For this review, take the finished solid that the model builds, in its own axes (mm). Face numbers are marked on the shaded views. A direction names the side the tool comes from. Round coordinates to 2 decimals unless told otherwise and drop trailing zeros. Order: outer loops, then holes, each group sorted by start corner. A loop starts at its lowest first (then second) coordinate and runs counter-clockwise, first axis right, second up. Notation, with made-up numbers: M 14,75 L 59,75 A27 cw 59,107 Z; hole C -5.5,7.5 d4. An arc over 180 degrees is marked long. Put each result on its own line as item: value.
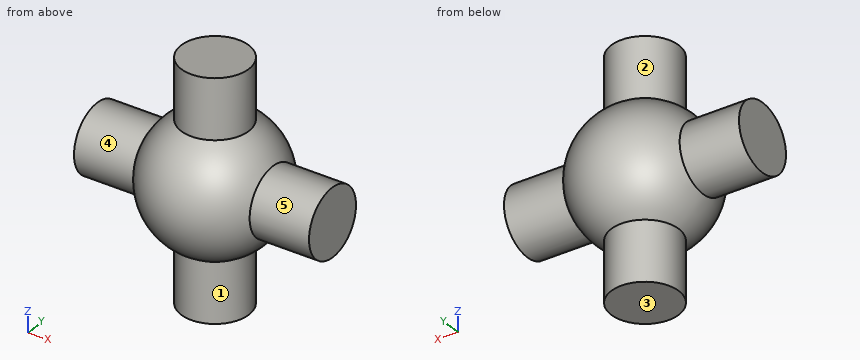
from build123d import *

# Parameters (mm, degrees)
SKETCH2_R           = 10
BOSS_EXTRUDE1_DEPTH = 35
SKETCH3_R           = 10
BOSS_EXTRUDE2_DEPTH = 35


with BuildPart() as part:
    # Sketch1 → Revolve1 (revolve)
    with BuildSketch(Plane(origin=(0, 0, 0), x_dir=(1, 0, 0), z_dir=(0, 1, 0))):
        with BuildLine():
            Line((0, 20), (0, -20))
            ThreePointArc((0, -20), (-20, 0), (0, 20))
        make_face()
    revolve(axis=Axis((0, 0, -20), (0, 0, 1)))



with BuildPart() as body_2:
    # Sketch2 → Boss-Extrude1 (new, symmetric)
    with BuildSketch(Plane.XY):
        Circle(SKETCH2_R)
    extrude(amount=BOSS_EXTRUDE1_DEPTH, both=True)


with BuildPart() as part_1:
    add(part.part)

    add(body_2.part)  # Boss-Extrude2 merges body 2
    # Sketch3 → Boss-Extrude2 (add, symmetric)
    with BuildSketch(Plane(origin=(0, 0, 0), x_dir=(0, 0, -1), z_dir=(1, 0, 0))):
        Circle(SKETCH3_R)
    extrude(amount=BOSS_EXTRUDE2_DEPTH, both=True)


solid = part_1.part
(1) Add section B-B on z = 0. Give the boundary of the cut face in (x, y).
A:
outline: M -35,-10 L -17.32,-10 A20 ccw 17.32,-10 L 35,-10 L 35,10 L 17.32,10 A20 ccw -17.32,10 L -35,10 Z
(2) Insertion check: pin 1 Ø12 at (y, z) = (6.5, -21.5) entering from +X; pin 2 Ø12 at (y, z) = (10.5, 25.5) entering from +X; pin 3 Ø1 at (x, y) = (20, 5.5) entering from -Z; pin 4 Ø8 at (x, y) = (13.5, -2) entering from +Z. Each pin has a flat end and moves straight along its axis. Give the tip position at first contact, or say it passes through.
A:
pin 1: stops at x = 11.36
pin 2: stops at x = 8.93
pin 3: stops at z = -8.66
pin 4: stops at z = 35
(3) Add section A-A on y = 0. Give the boundary of the cut face in (x, z).
A:
outline: M -35,-10 L -17.32,-10 A20 ccw -10,-17.32 L -10,-35 L 10,-35 L 10,-17.32 A20 ccw 17.32,-10 L 35,-10 L 35,10 L 17.32,10 A20 ccw 10,17.32 L 10,35 L -10,35 L -10,17.32 A20 ccw -17.32,10 L -35,10 Z
(4) For the marked faces 1, 2, 3, 4 and 5, list the 3-axis set-ups (+Z, -Z, +X, -X, +Y, -Y) from which the entire face can be reached by the end or side of a thin tool; tool diameter is ignored.
A:
face 1: -Z
face 2: +Z
face 3: -Z, +X, -X, +Y, -Y
face 4: -X
face 5: +X
(5) To check wall thickness, follow L1, parallel to X at y = 8, z = -10; L2, parallel to X at y = -15, z = -7.5; L3, parallel to Y at x = -4.5, z = -4. State the ranges of each line that lie inside material, in increasing order.
A:
L1: x = -15.36 to 15.36
L2: x = -10.9 to 10.9
L3: y = -19.07 to 19.07
(6) Add section D-D on z = 20. Give the boundary of the cut face in (x, y).
A:
outline: C 0,0 d20
(7) Add section C-C on x = 0. Give the boundary of the cut face in (y, z), then the cut area to 3 significant figures.
A:
outline: M -10,-35 L 10,-35 L 10,-17.32 A20 ccw 10,17.32 L 10,35 L -10,35 L -10,17.32 A20 ccw -10,-17.32 Z
area: 1,890 mm2
